Autodesk Inventor part; units mm, degrees
ref_plane "YZ Plane" through (0, 0, 0) normal (1, 0, 0) x (0, 1, 0)
ref_plane "XZ Plane" through (0, 0, 0) normal (0, 1, 0) x (-1, 0, 0)
ref_plane "XY Plane" through (0, 0, 0) normal (0, 0, 1) x (1, 0, 0)
sketch "スケッチ1" plane through (0, 0, 0) normal (0, 0, 1) x (1, 0, 0)
  line L0 (0, 0) -> (66.04, 0)
  line L1 (66.04, 0) -> (66.04, 2.54)
  line L2 (66.04, 2.54) -> (68.58, 5.08)
  line L3 (68.58, 5.08) -> (68.58, 37.846)
  line L4 (68.58, 37.846) -> (66.04, 40.386)
  line L5 (66.04, 40.386) -> (66.04, 51.816)
  line L6 (66.04, 51.816) -> (64.516, 53.34)
  line L7 (64.516, 53.34) -> (0, 53.34)
  line L8 (0, 53.34) -> (0, 0)
  dimension "d0" = 66.04
  dimension "d1" = 2.54
  dimension "d2" = 2.54
  dimension "d3" = 2.54
  dimension "d4" = 32.766
  dimension "d5" = 2.54
  dimension "d6" = 2.54
  dimension "d7" = 11.43
  dimension "d8" = 1.524
  dimension "d9" = 1.524
extrude "基板" add sketch "スケッチ1" along normal blind 1.8
sketch "スケッチ2" plane through (0, 0, 1.8) normal (0, 0, 1) x (1, 0, 0)
  circle A0 centre (13.97, 2.54) radius 1.5
  circle A1 centre (66.04, 7.62) radius 1.5
  circle A2 centre (66.04, 35.56) radius 1.5
  circle A3 centre (15.24, 50.8) radius 1.5
  point P0 (0, 0)
  dimension "d12" = 13.97
  dimension "d13" = 2.54
  dimension "d14" = 66.04
  dimension "d15" = 7.62
  dimension "d16" = 35.56
  dimension "d17" = 50.8
  dimension "d18" = 15.24
  dimension "d19" = 3
extrude "取付穴" cut sketch "スケッチ2" against normal blind 1.8
sketch "スケッチ4" plane through (0, 0, 1.8) normal (0, 0, 1) x (1, 0, 0)
  line L0 (11.595, 12.12) -> (-1.905, 12.12)
  line L1 (-1.905, 12.12) -> (-1.905, 3.12)
  line L2 (-1.905, 3.12) -> (11.595, 3.12)
  line L3 (11.595, 3.12) -> (11.595, 12.12)
  point P0 (0, 0)
  point P1 (-1.905, 7.62)
  point P2 (-1.905, 7.62)
  dimension "d22" = 7.62
  dimension "d23" = 1.905
  dimension "d24" = 13.5
  dimension "d25" = 9
extrude "電源ジャック" add sketch "スケッチ4" along normal blind 11
sketch "スケッチ5" plane through (0, 0, 12.8) normal (0, 0, 1) x (1, 0, 0)
  line L0 (11.595, 12.12) -> (1.595, 12.12)
  line L1 (1.595, 12.12) -> (1.595, 3.12)
  line L2 (1.595, 3.12) -> (11.595, 3.12)
  line L3 (11.595, 3.12) -> (11.595, 12.12)
  line L4 (11.595, 3.12) -> (11.595, 12.12)
  point P0 (0, 0)
  point P1 (11.595, 7.62)
  dimension "d28" = 9
  dimension "d29" = 10
extrude "押し出し4" cut sketch "スケッチ5" against normal blind 4.7
sketch "スケッチ6" plane through (0, 0, 8.1) normal (0, 0, 1) x (1, 0, 0)
  line L0 (11.595, 12.12) -> (1.595, 12.12)
  line L1 (1.595, 12.12) -> (1.595, 3.12)
  line L2 (1.595, 3.12) -> (11.595, 3.12)
  line L3 (11.595, 3.12) -> (11.595, 12.12)
  point P0 (0, 0)
extrude "押し出し5" add sketch "スケッチ6" along normal blind 4.5
fillet "フィレット1" radius 4.5 2 edges at (6.595, 3.12, 12.6) (6.595, 12.12, 12.6)
sketch "スケッチ7" plane through (0, 0, 1.8) normal (0, 0, 1) x (1, 0, 0)
  line L0 (-6.35, 44.1) -> (10.05, 44.1)
  line L1 (10.05, 44.1) -> (10.05, 32.1)
  line L2 (10.05, 32.1) -> (-6.35, 32.1)
  line L3 (-6.35, 32.1) -> (-6.35, 44.1)
  point P0 (0, 0)
  point P1 (-6.35, 38.1)
  point P2 (-6.35, 38.1)
  dimension "d35" = 6.35
  dimension "d36" = 38.1
  dimension "d37" = 16.4
  dimension "d38" = 12
extrude "USBジャック" add sketch "スケッチ7" along normal blind 11
sketch "スケッチ8" plane through (0, 0, 1.8) normal (0, 0, 1) x (1, 0, 0)
  line L0 (26.67, 3.81) -> (64.77, 3.81)
  line L1 (64.77, 3.81) -> (64.77, 1.27)
  line L2 (64.77, 1.27) -> (26.67, 1.27)
  line L3 (26.67, 1.27) -> (26.67, 3.81)
  point P0 (0, 0)
  point P1 (27.94, 2.54)
  point P2 (63.5, 2.54)
  point P3 (26.67, 2.54)
  dimension "d41" = 27.94
  dimension "d42" = 2.54
  dimension "d43" = 35.56
  dimension "d44" = 38.1
  dimension "d45" = 2.54
  dimension "d46" = 1.27
extrude "POWER ANALOG IN" add sketch "スケッチ8" along normal blind 8.5
sketch "スケッチ9" plane through (0, 0, 1.8) normal (0, 0, 1) x (1, 0, 0)
  line L0 (17.526, 51.51) -> (64.77, 51.51)
  line L1 (64.77, 51.51) -> (64.77, 48.97)
  line L2 (64.77, 48.97) -> (17.526, 48.97)
  line L3 (17.526, 48.97) -> (17.526, 51.51)
  point P0 (0, 0)
  point P1 (18.796, 50.24)
  point P2 (63.5, 50.24)
  point P3 (17.526, 50.24)
  dimension "d49" = 50.24
  dimension "d50" = 18.796
  dimension "d51" = 44.704
  dimension "d52" = 2.54
  dimension "d53" = 47.244
  dimension "d54" = 1.27
extrude "DIGITAL" add sketch "スケッチ9" along normal blind 8.5
properties part number "Arduino UNO"
The listing builds one solid part. Answer for the finished solid, in the listing's coordinates (mm). A direction names the side the tool comes from. Coordinates: 2 decimals unless noted, no trailing zeros. Loops run counter-clockwise (first coordinate to the right, second up) from the corner with the lowest first, then second, coordinate; pieces in that order, holes last. Notation, with made-up numbers: M 48.25,10.5 L 105.25,10.5 A13 cw 105.25,14.5 Z; hole C -38,30 d3. An arc over 180 degrees is marked long. Answer as a JSON object with one key per item and string values. Group by question number.
Item 1: Consider L1, parallel to Y at x = 8.5, z = 5.75; L2, parallel to Y at x = 60, z = 5; L3, parallel to Y at x = 13.97, z = 0.5. Determine where each line is inside the solid, lowest interval first.
Item 2: Determine the mould class of faces 1 (the face through (41, 48.97, 6)), 2 (the face through (17.526, 50, 6)), 3 (the face through (65.289, 52.567, 0.887)), 4 (the face through (12.47, 2.61, 0.91)) for opening direction X: +X half, -X half, draft (parallel to the pull), parting line (faces both ways), or undercut.
Item 3: Which of the six approach directions +Z, -Z, +X, -X, +Y, -Y give full straight-line access (tool end or side, diameter ignored) to faces 5 (the face through (26.67, 3, 6)), 6 (the face through (2, 32.1, 7)), 7 (the face through (41, 51.51, 6)), 8 (the face through (66.04, 46, 1))?
Item 4: Section A-A (z = 2.75) is taken. Write down the section's boundary in (x, y) (3 decimals), and give its area (3 significant figures).
Item 5: Section D-D (y = 22) is taken. Write down the section's boundary in (x, z), and give its area (3 significant figures).
Item 6: Each of these flat-tipped pins is pushed along its axis until it touches: P1, Ø8, axis at x = 20.5, y = 39.5, coming from the -Z side; P2, Ø3, axis at x = 35, y = 51, coming from the +Z side; P3, Ø0.9, axis at y = 17, z = 1, coming from the -X side; P4, Ø8, axis at x = 34.5, y = 38.5, coming from the +Z side. Where does it stop, or does it pass through?
Item 7: Section C-C (y = 35.56) is taken. Write down the section's boundary in (x, z), and give its area (3 significant figures).
Solved:
{
 "1": {"L1": "y = 3.12 to 12.12, 32.1 to 44.1", "L2": "y = 1.27 to 3.81, 48.97 to 51.51", "L3": "y = 0 to 1.04, 4.04 to 50, 51.6 to 53.34"},
 "2": {"face 1": "draft", "face 2": "-X half", "face 3": "+X half", "face 4": "undercut"},
 "3": {"face 5": "+Z, -Y", "face 6": "+Z, +X, -X", "face 7": "+Z, +X, -X, +Y", "face 8": "+Z, -Z, +X, +Y"},
 "4": {"outline": "M -6.35,32.1 L 10.05,32.1 L 10.05,44.1 L -6.35,44.1 Z; M -1.905,3.12 L 11.595,3.12 L 11.595,12.12 L -1.905,12.12 Z; M 17.526,48.97 L 64.77,48.97 L 64.77,51.51 L 17.526,51.51 Z; M 26.67,1.27 L 64.77,1.27 L 64.77,3.81 L 26.67,3.81 Z", "area": "535 mm2"},
 "5": {"outline": "M 0,0 L 68.58,0 L 68.58,1.8 L 0,1.8 Z", "area": "123 mm2"},
 "6": {"P1": "stops at z = 0", "P2": "stops at z = 10.3", "P3": "stops at x = 0", "P4": "stops at z = 1.8"},
 "7": {"outline": "M -6.35,1.8 L 0,1.8 L 0,0 L 64.54,0 L 64.54,1.8 L 10.05,1.8 L 10.05,12.8 L -6.35,12.8 Z; M 67.54,0 L 68.58,0 L 68.58,1.8 L 67.54,1.8 Z", "area": "298 mm2"}
}
